from build123d import *

# Parameters (mm, degrees)
SKETCH1_W           = 99
SKETCH1_H           = 63
BOSS_EXTRUDE1_DEPTH = 22
SKETCH5_W           = 10.2
SKETCH5_H           = 63
BOSS_EXTRUDE3_DEPTH = 1
SKETCH7_R           = 1.9
CUT_EXTRUDE2_DEPTH  = 1
SKETCH8_R           = 5.461
BOSS_EXTRUDE4_DEPTH = 1.27
SKETCH9_R           = 3.556
SKETCH9_R_2         = 2.032
BOSS_EXTRUDE5_DEPTH = 0.762
FILLET1_R           = 1
CHAMFER1_SIZE       = 1
SKETCH10_R          = 2.27
CUT_EXTRUDE3_DEPTH  = 20
SKETCH11_R          = 2.413
CUT_EXTRUDE4_DEPTH  = 0.762
FILLET3_R           = 1.27


with BuildPart() as part:
    # Sketch1 → Boss-Extrude1 (new body)
    with BuildSketch(Plane(origin=(0, 0, 0), x_dir=(1, 0, 0), z_dir=(0, 1, 0))):
        with Locations((49.5, 31.5)):
            Rectangle(SKETCH1_W, SKETCH1_H)
    extrude(amount=BOSS_EXTRUDE1_DEPTH)

    # Sketch5 → Boss-Extrude3 (add)
    with BuildSketch(Plane.XZ):
        with Locations((-5.1, -31.5)):
            Rectangle(SKETCH5_W, SKETCH5_H)
        with Locations((104.1, -31.5)):
            Rectangle(SKETCH5_W, SKETCH5_H)
    extrude(amount=-BOSS_EXTRUDE3_DEPTH)

    # Sketch7 → Cut-Extrude2 (cut)
    with BuildSketch(Plane(origin=(0, 1, 0), x_dir=(1, 0, 0), z_dir=(0, 1, 0))):
        with Locations(Location((104.1, 5.71, 0), (0, 0, 270))):
            Circle(SKETCH7_R)
        with Locations(Location((-5.1, 5.71, 0), (0, 0, 270))):
            Circle(SKETCH7_R)
        with BuildLine():
            Line((102.15, 57.75), (102.15, 54.662235902))
            ThreePointArc((102.15, 54.662235902), (104.1, 48.7), (106.05, 54.662235902))
            Line((106.05, 54.662235902), (106.05, 57.75))
            ThreePointArc((106.05, 57.75), (104.1, 59.7), (102.15, 57.75))
        make_face()
        with BuildLine():
            Line((-7.05, 57.75), (-7.05, 54.662235902))
            ThreePointArc((-7.05, 54.662235902), (-5.1, 48.7), (-3.15, 54.662235902))
            Line((-3.15, 54.662235902), (-3.15, 57.75))
            ThreePointArc((-3.15, 57.75), (-5.1, 59.7), (-7.05, 57.75))
        make_face()
    extrude(amount=-CUT_EXTRUDE2_DEPTH, mode=Mode.SUBTRACT)

    # Sketch8 → Boss-Extrude4 (add)
    with BuildSketch(Plane.XY):
        with Locations(Location((15.24, 11.5, 0), (0, 0, 180))):
            Circle(SKETCH8_R)
        with Locations(Location((83.76, 11.5, 0), (0, 0, 180))):
            Circle(SKETCH8_R)
    extrude(amount=BOSS_EXTRUDE4_DEPTH)

    # Sketch9 → Boss-Extrude5 (add)
    # profile 1 of 2: a face of its own
    with BuildSketch(Plane.XY.offset(1.27)):
        with Locations(Location((15.24, 11.5, 0), (0, 0, 180))):
            Circle(SKETCH9_R)
        with Locations(Location((15.24, 11.5, 0), (0, 0, 180))):
            Circle(SKETCH9_R_2, mode=Mode.SUBTRACT)
    # profile 2 of 2: a face of its own
    with BuildSketch(Plane.XY.offset(1.27)):
        with Locations(Location((83.76, 11.5, 0), (0, 0, 180))):
            Circle(SKETCH9_R)
        with Locations(Location((83.76, 11.5, 0), (0, 0, 180))):
            Circle(SKETCH9_R_2, mode=Mode.SUBTRACT)
    extrude(amount=BOSS_EXTRUDE5_DEPTH)

    # Fillet1
    fillet1_edges = [part.edges().sort_by_distance(p)[0] for p in [
        (20.701, 11.5, 1.27),
        (89.221, 11.5, 1.27),
    ]]
    fillet(fillet1_edges, radius=FILLET1_R)

    # Chamfer1
    # the kernel refuses this chamfer: 1 mm, written as the material it takes off along each edge
    with BuildSketch(Plane(origin=(83.76, 11.5, 2.032), x_dir=(-1, 0, 0), z_dir=(0, 1, 0))) as chamfer1_piece_1_section:
        Polygon((2.032 + CHAMFER1_SIZE, 0), (2.032, -CHAMFER1_SIZE), (2.032, 0), align=None)
    chamfer1_piece_1 = revolve(axis=Axis((83.76, 11.5, 2.032), (0, 0, 1)), mode=Mode.PRIVATE)
    chamfer1_piece_1 = split(chamfer1_piece_1, bisect_by=Plane(origin=(86.411200438, 11.5, 1.27), z_dir=(0, 0, 1)), keep=Keep.TOP, mode=Mode.PRIVATE)
    add(chamfer1_piece_1, mode=Mode.SUBTRACT)
    with BuildSketch(Plane(origin=(15.24, 11.5, 2.032), x_dir=(-1, 0, 0), z_dir=(0, 1, 0))) as chamfer1_piece_2_section:
        Polygon((2.032 + CHAMFER1_SIZE, 0), (2.032, -CHAMFER1_SIZE), (2.032, 0), align=None)
    chamfer1_piece_2 = revolve(axis=Axis((15.24, 11.5, 2.032), (0, 0, 1)), mode=Mode.PRIVATE)
    chamfer1_piece_2 = split(chamfer1_piece_2, bisect_by=Plane(origin=(17.891200438, 11.5, 1.27), z_dir=(0, 0, 1)), keep=Keep.TOP, mode=Mode.PRIVATE)
    add(chamfer1_piece_2, mode=Mode.SUBTRACT)

    # Sketch10 → Cut-Extrude3 (cut)
    with BuildSketch(Plane.XY.offset(1.27)):
        with Locations((15.24, 11.5)):
            Circle(SKETCH10_R)
        with Locations((83.76, 11.5)):
            Circle(SKETCH10_R)
    extrude(amount=-CUT_EXTRUDE3_DEPTH, mode=Mode.SUBTRACT)

    # Sketch11 → Cut-Extrude4 (cut)
    with BuildSketch(Plane.XY):
        with Locations((34.26, 11.5)):
            Circle(SKETCH11_R)
        with Locations((64.74, 11.5)):
            Circle(SKETCH11_R)
    extrude(amount=-CUT_EXTRUDE4_DEPTH, mode=Mode.SUBTRACT)

    # Sketch13 → Revolve1 (revolve)
    with BuildSketch(Plane(origin=(34.26, 11.5, -0.762), x_dir=(1, 0, 0), z_dir=(0, 1, 0))):
        with BuildLine():
            Line((0, 2.159), (0, -2.159))
            ThreePointArc((0, -2.159), (2.159, 0), (0, 2.159))
        make_face()
    revolve(axis=Axis((34.26, 11.5, -2.921), (0, 0, -1)))

    # Sketch15 → Revolve2 (revolve)
    with BuildSketch(Plane(origin=(34.26, 11.5, -0.762), x_dir=(1, 0, 0), z_dir=(0, 1, 0))):
        with BuildLine():
            Line((30.48, -2.159), (30.48, 2.159))
            ThreePointArc((30.48, 2.159), (32.639, 0), (30.48, -2.159))
        make_face()
    revolve(axis=Axis((64.74, 11.5, -2.921), (0, 0, -1)))

    # Fillet3
    fillet3_edges = [part.edges().sort_by_distance(p)[0] for p in [
        (99, 22, -31.5),
        (49.5, 22, -63),
        (0, 22, -31.5),
        (99, 11.5, -63),
        (99, 11.5, 0),
        (0, 11.5, 0),
        (49.5, 22, 0),
    ]]
    fillet(fillet3_edges, radius=FILLET3_R)


solid = part.part
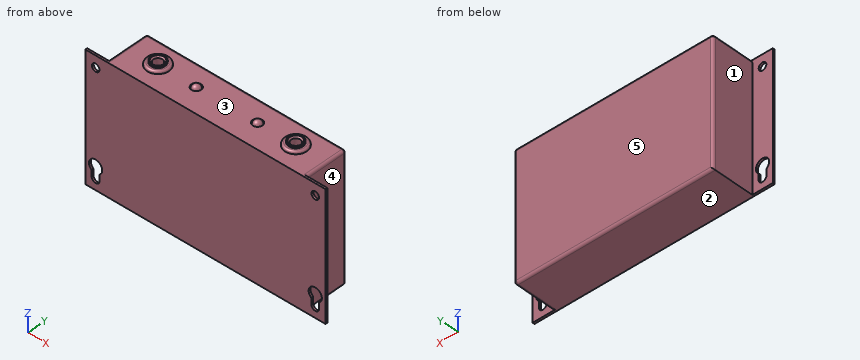
Input: part model. Units: mm. Frame: model coordinates. Face numbers are marked on the shaded views. A direction names the side the tool comes from. Coordinates: 2 decimals unless noted, no trailing zeros. Loops run counter-clockwise (first coordinate to the right, second up) from the corner with the lowest first, then second, coordinate; pieces in that order, holes last.
Q1. Cut plane C-C (z = -24.5). Output: boundary loops of the cut face in (x, y), then the cut area to 3 significant figures.
Q2. Material intervals for line 1 (X direction, y = 14.25, z = -12); line 2 (Y direction, x = -5, z = -45.5); line 3 (Y direction, x = 83.76, z = -4.5), sorted ascending.
Q3. Cut plane A-A (z = -52). Output: boundary loops of the cut face in (x, y).
Q4. Contact query for flat-ended pins moving along their axis: pin 1 (12 mm diameter, centred on y = 9.5, z = -48.5, fed in from -X); pin 2 (4 mm diameter, centred on x = 65.5, y = 12.5, fed in from +Z); pin 3 (10.5 mm diameter, centred on x = 24, y = 13.5, fed in from +Z); pin 4 (5 mm diameter, centred on x = 83, y = 10.5, fed in from +Z). Output: stop coordinate, or through.
Q5. Draft query along X for the marked faces 1, 2 and 3. Return one class per face: +X half, -X half, draft (parallel to the pull), parting line (faces both ways), or undercut.
Q6. Cut plane D-D (y = 18.75). Output: boundary loops of the cut face in (x, z), then the cut area to 3 significant figures.
Q7. Cut plane B-B (x = -5.1). Output: boundary loops of the cut face in (y, z).
Q8. Set-up query: the marked faces 4 and 5. Return all of +Z, -Z, +X, -X, +Y, -Y with unobstructed straight access to the full face (end or side cutting, diameter ignored); none if empty.
Working result:
1. outline: (-10.2, 0) - (109.2, 0) - (109.2, 1) - (99, 1) - (99, 20.73) arc R1.27 ccw to (97.73, 22) - (1.27, 22) arc R1.27 ccw to (0, 20.73) - (0, 1) - (-10.2, 1) - close
1. area: 2,200 mm2
2. line 1: x = 0 to 99
2. line 2: y = 0 to 1
2. line 3: y = 0 to 9.23, 13.77 to 22
3. outline: (-10.2, 0) - (-8.4, 0) - (-8.4, 1) - (-10.2, 1) - close; (-1.8, 0) - (100.8, 0) - (100.8, 1) - (99, 1) - (99, 20.73) arc R1.27 ccw to (97.73, 22) - (1.27, 22) arc R1.27 ccw to (0, 20.73) - (0, 1) - (-1.8, 1) - close; (107.4, 0) - (109.2, 0) - (109.2, 1) - (107.4, 1) - close
4. pin 1: stops at x = 0
4. pin 2: stops at z = 1.4
4. pin 3: stops at z = 1.27
4. pin 4: stops at z = 2.03
5. face 1: -X half
5. face 2: draft
5. face 3: undercut
6. outline: (0, -63) - (97.73, -63) arc R1.27 ccw to (99, -61.73) - (99, -1.27) arc R1.27 ccw to (97.73, 0) - (1.27, 0) arc R1.27 ccw to (0, -1.27) - close
6. area: 6,240 mm2
7. outline: (0, -63) - (1, -63) - (1, -59.7) - (0, -59.7) - close; (0, -48.7) - (1, -48.7) - (1, -7.61) - (0, -7.61) - close; (0, -3.81) - (1, -3.81) - (1, 0) - (0, 0) - close
8. face 4: +Z, -Z, +X, +Y
8. face 5: +Z, -Z, +X, -X, +Y
